from build123d import *
from build123d import SkipClean  # not in build123d's __all__

# Parameters (mm, degrees)
F0_R     = 80
F0_R_2   = 6
F1_DEPTH = 1
F3_DEPTH = 1


with BuildPart() as f1:
    # F0 (on Top) → F1 (new body)
    with BuildSketch(Plane.XY):
        Circle(F0_R)
        Circle(F0_R_2, mode=Mode.SUBTRACT)
    extrude(amount=F1_DEPTH)

    # F2 (on face) → F3 (join)
    with BuildSketch(Plane.XY.offset(1)):
        with BuildLine():
            ThreePointArc((80, 0), (56.5685424949, 56.5685424949), (0, 80))
            Line((0, 80), (0, 52.1204726901))
            Line((0, 52.1204726901), (-5.8869810823, 57.0602363451))
            Line((-5.8869810823, 57.0602363451), (-5.8869810823, 32.0602363451))
            Line((-5.8869810823, 32.0602363451), (0, 37))
            Line((0, 37), (0, 6))
            ThreePointArc((0, 6), (4.2426406871, 4.2426406871), (6, 0))
            Line((6, 0), (37, 0))
            Line((37, 0), (32.0602363451, 5.8869810823))
            Line((32.0602363451, 5.8869810823), (57.0602363451, 5.8869810823))
            Line((57.0602363451, 5.8869810823), (52.1204726901, 0))
            Line((52.1204726901, 0), (80, 0))
        make_face()
    with SkipClean():  # cleaning this boolean's faces spoils the solid; the shape is the same uncleaned
        extrude(amount=F3_DEPTH)


solid = f1.part
Build history of the part. All positions in model axes, mm. Give positions to 0.01 mm unless a question says otherwise; leave off trailing zeros. Order: outer loops, then holes, each group sorted by start corner. A loop starts at its lowest first (then second) coordinate and runs counter-clockwise, first axis right, second up. Notation, with made-up numbers: M -6,49 L 46,49 A27 ccw 46,73 Z; hole C 88.25,13 d7. An arc over 180 degrees is marked long. Use one line per item in the form item = value.
Q1. Wall check: probe 1 along Y at (x, z) = (0, 0.65); probe 2 along Z at (x, y) = (24, -33). Give the ranges that are in metal, low to high.
Conclusion:
probe_1 = -80 to -6, 6 to 80
probe_2 = 0 to 1
Q2. Slice it at D-D, the plane x = 28. Write the cut outline in (y, z).
Conclusion:
outline = M -74.94,0 L 74.94,0 L 74.94,2 L 0,2 L 0,1 L -74.94,1 Z
Q3. Pin check, flat tips, straight feed: P1, Ø3, axis at x = 47, y = -55, coming from the -Z side; P2, Ø0.5, axis at y = 65.5, z = 1.5, coming from the -X side; P3, Ø10, axis at x = -12.5, y = -29.5, coming from the +Z side; P4, Ø0.8, axis at x = 16, z = 1.5, coming from the -Y side. Stop position of each tip, or through.
Conclusion:
P1 = 0
P2 = 0
P3 = 1
P4 = 0
Q4. Slice it at B-B, the plane z = 0.65. Write the cut outline in (x, y).
Conclusion:
outline = C 0,0 d160; hole C 0,0 d12
Q5. Slice it at A-A, the plane y = 3.5. Write the cut outline in (x, z), and give its area (3 significant figures).
Conclusion:
outline = M -79.92,0 L -4.87,0 L -4.87,1 L -79.92,1 Z; M 4.87,0 L 79.92,0 L 79.92,2 L 55.06,2 L 55.06,1 L 34.06,1 L 34.06,2 L 4.87,2 Z
area = 204 mm2
Q6. Pull direction X, two halves, no side cores. Call faces 1 (the flat face through (34.565, 2.902, 1.493)), 2 (the flat face through (17, 1, 0)): released by +X, released by -X, zero draft, split by the parting line, or undercut.
Conclusion:
face_1 = undercut
face_2 = zero draft
Q7. Slice it at C-C, the plane y = 22. Write the cut outline in (x, z), and give its area (3 significant figures).
Conclusion:
outline = M -76.92,0 L 76.92,0 L 76.92,2 L 0,2 L 0,1 L -76.92,1 Z
area = 231 mm2
